Can you work these out from the model? Positions are in its coordinate system, mm. A direction names the side the tool comes from. Give positions to 0.01 mm unless a question says otherwise; leave off trailing zeros. Write each loop counter-clockwise with the first axis right and the second up, starting at its lowest first coordinate (ties: lowest second). Pieces come first, ordered by that corner, then holes. Notation, with made-up numbers: (-3, 28.25) - (12, 28.25) arc R16 ccw to (12, 45.25) - close; hole circle Ø4 at (64.25, 4). An arc over 180 degrees is marked (long way). Return JSON: item names as keys, results as strings. Group by question number.
from build123d import *

# Parameters (mm, degrees)
SALIENTE_EXTRUIR1_DEPTH = 11.7
CROQUIS3_R              = 3.75
SALIENTE_EXTRUIR2_DEPTH = 5.4
CROQUIS5_R              = 3
SALIENTE_EXTRUIR3_DEPTH = 5.4


with BuildPart() as part:
    # Croquis2 → Saliente-Extruir1 (new, symmetric)
    with BuildSketch(Plane.XY):
        Polygon((-21.3, 7.12), (-21.3, 0), (-2.375, 0), (-2.375, -17.1), (2.375, -17.1), (2.375, 0), (21.3, 0), (21.3, 7.12), align=None)
    extrude(amount=SALIENTE_EXTRUIR1_DEPTH, both=True)

    # Croquis3 → Saliente-Extruir2 (add)
    with BuildSketch(Plane(origin=(0, 7.12, 0), x_dir=(1, 0, 0), z_dir=(0, 1, 0))):
        with Locations((-9.3, 0)):
            Circle(CROQUIS3_R)
        with Locations((9.3, 0)):
            Circle(CROQUIS3_R)
    extrude(amount=SALIENTE_EXTRUIR2_DEPTH)

    # Croquis5 → Saliente-Extruir3 (add)
    with BuildSketch(Plane(origin=(2.375, 0, 0), x_dir=(0, 0, -1), z_dir=(1, 0, 0))):
        with Locations(Location((0, -8.55, 0), (0, 0, 180))):
            Circle(CROQUIS5_R)
    saliente_extruir3 = extrude(amount=SALIENTE_EXTRUIR3_DEPTH)

    # Simetría1: Saliente-Extruir3 across plane
    add(saliente_extruir3.mirror(Plane(origin=(0, 0, 0), x_dir=(0, 0, 1), z_dir=(1, 0, 0))))


solid = part.part
1) I need wall thicknesses on line 1 along Y through (x, z) = (-3.5, -8); line 2 along X through (y, z) = (-11.25, 8.5) (3 decimals); line 3 along Y through (x, z) = (-12, -0.5). Which ranges of each line are inside material? Lowest first, please.
2) On a 3-axis mill with a long thin cutter (end or side, diameter ignored), from which of +Z, -Z, +X, -X, +Y, -Y can I reach the whole of each face in a straight line? I mean faces 4 (the face through (-7.775, -9, 0)), 5 (the face through (2.375, -11, 3)), 6 (the face through (-5.836, 9.782, 1.436)), 7 (the face through (-2.375, -7, 3)), 8 (the face through (7.775, -9, 0)). Say none if no direction works.
3) We'd pull the mould along Y, two halves only. Please class faces 1 (the face through (0, -17.1, 0)), 2 (the face through (-5.04, -11.08, 1.61)), 3 (the face through (21.3, 4, 0)): pulls with the +Y half, pulls with the -Y half, needs draft (parallel to the pull), parting line crosses it, or undercut.
4) Will these pins go through, and if not, where does the flat tip stop? pin 1 Ø1.5 at (x, z) = (6, -0.5) entering from -Y; pin 2 Ø4 at (x, z) = (1, 9) entering from +Y; pin 3 Ø6.5 at (y, z) = (-10, -0.5) entering from -X (3 decimals).
5) Imagine slicing it at A-A, the plane x = -9.3. Write out the boundary of the cut face in (y, z).
6) Imagine slicing it at D-D, the plane y = 10. Write out the boundary of the cut face in (x, z).
7) Imagine slicing it at C-C, the plane y = -8.55. Write out the boundary of the cut face in (x, z) (3 decimals), and give its area (3 significant figures).
8) Imagine slicing it at B-B, the plane z = 9. Write out the boundary of the cut face in (x, y) (3 decimals), and give its area (3 significant figures).
Resolved:
{
 "1": {"line 1": "0 to 7.12", "line 2": "-2.375 to 2.375", "line 3": "0 to 12.52"},
 "2": {"face 4": "+Z, -Z, -X, -Y", "face 5": "+X", "face 6": "+Y", "face 7": "-X", "face 8": "+Z, -Z, +X, -Y"},
 "3": {"face 1": "pulls with the -Y half", "face 2": "undercut", "face 3": "needs draft"},
 "4": {"pin 1": "y = -11.55", "pin 2": "y = 7.12", "pin 3": "x = -7.775"},
 "5": {"outline": "(0, -11.7) - (7.12, -11.7) - (7.12, -3.75) - (12.52, -3.75) - (12.52, 3.75) - (7.12, 3.75) - (7.12, 11.7) - (0, 11.7) - close"},
 "6": {"outline": "circle Ø7.5 at (-9.3, 0); circle Ø7.5 at (9.3, 0)"},
 "7": {"outline": "(-7.775, -3) - (-2.375, -3) - (-2.375, -11.7) - (2.375, -11.7) - (2.375, -3) - (7.775, -3) - (7.775, 3) - (2.375, 3) - (2.375, 11.7) - (-2.375, 11.7) - (-2.375, 3) - (-7.775, 3) - close", "area": "176 mm^2"},
 "8": {"outline": "(-21.3, 0) - (-2.375, 0) - (-2.375, -17.1) - (2.375, -17.1) - (2.375, 0) - (21.3, 0) - (21.3, 7.12) - (-21.3, 7.12) - close", "area": "385 mm^2"}
}
